Geometry: see drawing. Coordinates: mm, zero at the bounding-box minimum. A direction names the side the tool comes from. Coordinates: 2 decimals unless noted, no trailing zeros. Write each loop counter-clockwise with the first axis right and the second up, starting at its lowest first coordinate (ties: lowest second). Pieces come first, ordered by that corner, then holes. Notation, with made-up numbers: M -33.5,50.25 L -14.5,50.25 A14 cw -14.5,68.25 Z; hole C -23,71.5 d11. An arc over 180 degrees is marked long. Answer as CSV lines item,"result". Start each with the question number.
1. Reachability of the marked faces 4 and 5 from +Z, -Z, +X, -X, +Y, -Y: full face, straight path, thin tool, end or side. Return the list, or none.
2. Contact query for a flat-ended pin moving along its axis: pin 1 Ø3 at (x, y) = (6, 14) entering from -Z. Output: stop coordinate, or through.
3. Line query: probe 1 along Y at (x, z) = (3, 5.5); probe 2 along Y at (x, z) = (5.25, 9.5); probe 3 along Z at (x, y) = (2, 19). Output: solid intervals per line, ascending. Write a range as [from, to].
4. Section A-A on x = 2.75. Return the cut outline in (y, z).
5. Mould query, pull axis X, two halves, no side actions, for the marked faces 1, 2 and 3. Classes: pulls with the +X half, pulls with the -X half, needs draft (parallel to the pull), parting line crosses it, or undercut.
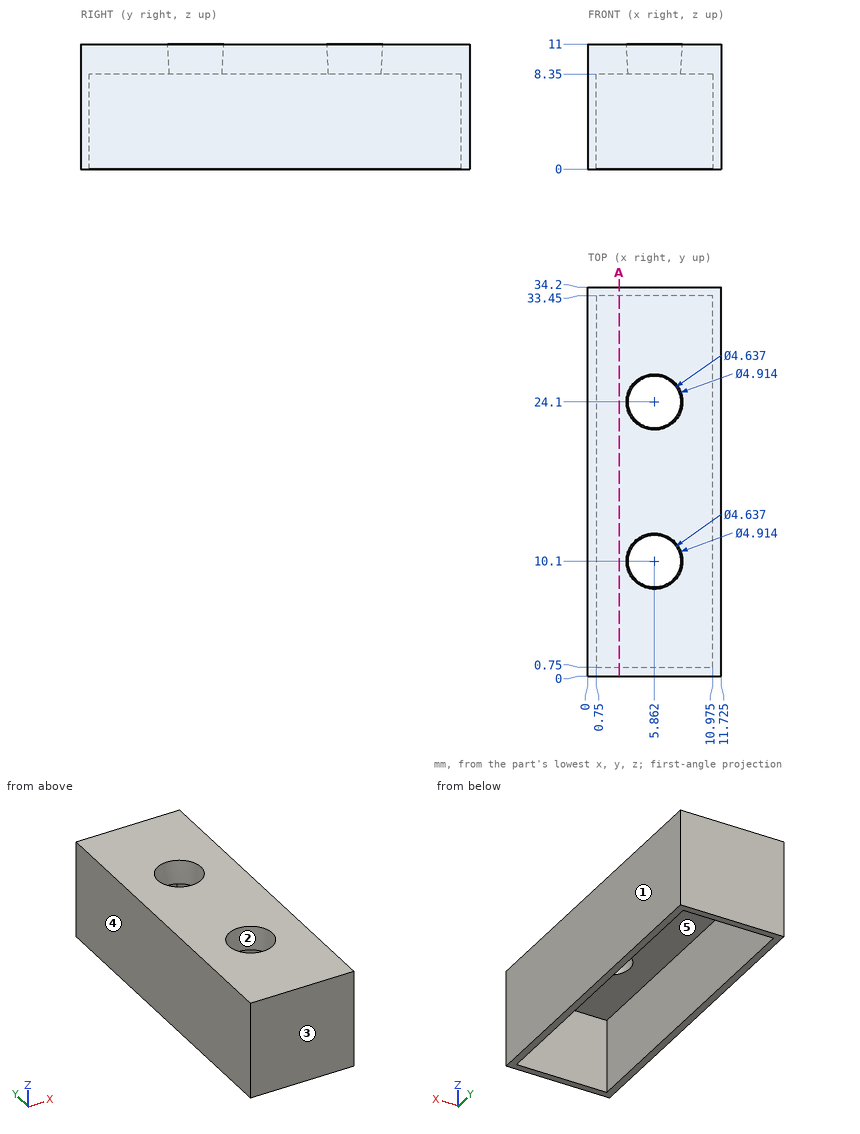
Values:
1,face 4,"+Z, -Z, -X, +Y, -Y"
1,face 5,"-Z"
2,pin 1,"z = 8.35"
3,probe 1,"[0, 0.75], [33.45, 34.2]"
3,probe 2,"[0, 7.8], [12.4, 21.8], [26.4, 34.2]"
3,probe 3,"[8.35, 11]"
4,outline,"M 0,0 L 0.75,0 L 0.75,8.35 L 33.45,8.35 L 33.45,0 L 34.2,0 L 34.2,11 L 0,11 Z"
5,face 1,"pulls with the +X half"
5,face 2,"undercut"
5,face 3,"needs draft"
